Verification items for the finished model (mm, model axes). A direction names the side the tool comes from. Round coordinates to 2 decimals unless told otherwise and drop trailing zeros. Order: outer loops, then holes, each group sorted by start corner. A loop starts at its lowest first (then second) coordinate and runs counter-clockwise, first axis right, second up. Notation, with made-up numbers: M 47,-23.75 L 62,-23.75 A13 cw 62,-5.75 Z; hole C 62.5,-17.75 d9. An arc over 180 degrees is marked long. One line per item, written item: value. Start each with the question number.
from build123d import *

# Parameters (mm, degrees)
BOSS_EXTRU_1_DEPTH      = 2
CONG_1_R                = 10
ENL_V_MAT_EXTRU_1_DEPTH = 2
CONG_2_R                = 10
ESQUISSE3_R             = 1.6
ENL_V_MAT_EXTRU_2_DEPTH = 10


with BuildPart() as part:
    # Esquisse1 → Boss.-Extru.1 (new body)
    with BuildSketch(Plane.XY):
        Polygon((-40.879571388, 34.615718895), (81.042798068, 34.615718895), (104.193503713, 7.025782272), (38.617977526, -93.674532757), (1.545249154, -93.674532757), (-64.030277033, 7.025782272), align=None)
    extrude(amount=BOSS_EXTRU_1_DEPTH)

    # Congé1
    cong_1_edges = [part.edges().sort_by_distance(p)[0] for p in [
        (-40.879571388, 34.615718895, 1),
        (81.042798068, 34.615718895, 1),
        (104.193503713, 7.025782272, 1),
        (38.617977526, -93.674532757, 1),
        (1.545249154, -93.674532757, 1),
        (-64.030277033, 7.025782272, 1),
    ]]
    fillet(cong_1_edges, radius=CONG_1_R)

    # Esquisse2 → Enlèv. mat.-Extru.1 (cut)
    with BuildSketch(Plane.XY.offset(2)):
        Polygon((-36.216494806, 24.615718895), (-51.607204261, 6.27378561), (6.96667711, -83.674532757), (33.19654957, -83.674532757), (91.770430941, 6.27378561), (76.379721487, 24.615718895), align=None)
    extrude(amount=-ENL_V_MAT_EXTRU_1_DEPTH, mode=Mode.SUBTRACT)

    # Congé2
    cong_2_edges = [part.edges().sort_by_distance(p)[0] for p in [
        (-36.216494806, 24.615718895, 1),
        (76.379721487, 24.615718895, 1),
        (91.770430941, 6.27378561, 1),
        (33.19654957, -83.674532757, 1),
        (6.96667711, -83.674532757, 1),
        (-51.607204261, 6.27378561, 1),
    ]]
    fillet(cong_2_edges, radius=CONG_2_R)

    # Esquisse3 → Enlèv. mat.-Extru.2 (cut)
    with BuildSketch(Plane.XY.offset(2)):
        with Locations((20.08161334, -91.058073416)):
            Circle(ESQUISSE3_R)
        with Locations((-28.872824595, -42.931783887)):
            Circle(ESQUISSE3_R)
        with Locations((20.08161334, 32.415718895)):
            Circle(ESQUISSE3_R)
        with Locations((90.076701777, 20.426939275)):
            Circle(ESQUISSE3_R)
        with Locations((69.036051275, -42.931783887)):
            Circle(ESQUISSE3_R)
        with Locations((-49.913475097, 20.426939275)):
            Circle(ESQUISSE3_R)
    extrude(amount=-ENL_V_MAT_EXTRU_2_DEPTH, mode=Mode.SUBTRACT)


solid = part.part
1. Section check C-C (x = -7.5). Record the cut outline in (y, z).
2. Scan lines: line 1 along X through (y, z) = (-14.5, 1.85); line 2 along X through (y, z) = (-78.5, 0.75); line 3 along X through (y, z) = (20, 0.7). Record each from-to range of solid material in increasing order.
3. Draft check along Y on faces 3 (the face through (2.262, -92.499, 1.014)), 4 (the face through (61.58, -40.09, 1.01)), 5 (the face through (91.63, 22, 0.99)). Enter one of: released by +Y, released by -Y, zero draft, split by the parting line, or undercut.
4. Section check B-B (z = 0.55). Give the number of separate pieces and of enclosed holes in the cut face, and give its area (3 significant figures).
5. Tool access check on faces 1 (the face through (83.25, 16.43, 1.01)), 2 (the face through (71.27, -43.53, 0.99)). Record the directions out of +Z, -Z, +X, -X, +Y, -Y that give a thin tool (end or side, any length) a straight path to the whole face; none if there is none.
6. Depth check by flat-ended pin: pin 1 (2.5 mm diameter, centred on x = -49.91, y = 20.43, fed in from -Z). Enter the tip coordinate at first touch or a pass-through.
7. Section check A-A (y = 16.5). Record the cut outline in (x, z).
Geometry check:
1. outline: M -79.78,0 L -61.46,0 L -61.46,2 L -79.78,2 Z; M 24.62,0 L 34.62,0 L 34.62,2 L 24.62,2 Z
2. line 1: x = -50.01 to -38.08, 78.24 to 90.18
2. line 2: x = -8.34 to 3.6, 36.57 to 48.5
2. line 3: x = -53.14 to -51.46, -48.37 to -40.09, 80.25 to 88.53, 91.62 to 93.31
3. face 3: released by -Y
3. face 4: undercut
3. face 5: released by +Y
4. separate pieces: 1
4. enclosed holes: 7
4. area: 4,320 mm²
5. face 1: +Z, -Z
5. face 2: +Z, -Z, +X, -Y
6. pin 1: passes through
7. outline: M -56.08,0 L -43.03,0 L -43.03,2 L -56.08,2 Z; M 83.19,0 L 96.24,0 L 96.24,2 L 83.19,2 Z
